```python
from build123d import *

# Parameters (mm, degrees)
F0_R      = 5
F1_DEPTH  = 35
F2_R      = 11.5
F3_DEPTH  = 78
F4_R      = 15
F5_DEPTH  = 25
F6_R      = 5
F7_DEPTH  = 25
F9_W      = 40
F9_H      = 8
F10_DEPTH = 4


with BuildPart() as f1:
    # F0 (on Right) → F1 (new body)
    with BuildSketch(Plane.YZ):
        Circle(F0_R)
    extrude(amount=F1_DEPTH)

    # F2 (on face) → F3 (join)
    with BuildSketch(Plane(origin=(0, 0, 0), x_dir=(0, -1, 0), z_dir=(-1, 0, 0))):
        Circle(F2_R)
    extrude(amount=F3_DEPTH)

    # F4 (on face) → F5 (join)
    with BuildSketch(Plane(origin=(-78, 0, 0), x_dir=(0, -1, 0), z_dir=(-1, 0, 0))):
        Circle(F4_R)
    extrude(amount=F5_DEPTH)

    # F6 (on face) → F7 (join)
    with BuildSketch(Plane(origin=(-103, 0, 0), x_dir=(0, -1, 0), z_dir=(-1, 0, 0))):
        Circle(F6_R)
    extrude(amount=F7_DEPTH)

    # F9 (on offset) → F10 (cut)
    with BuildSketch(Plane.XY.offset(11.5)):
        with Locations((-41.2988585503, 0)):
            Rectangle(F9_W, F9_H)
    extrude(amount=-F10_DEPTH, mode=Mode.SUBTRACT)


solid = f1.part
```
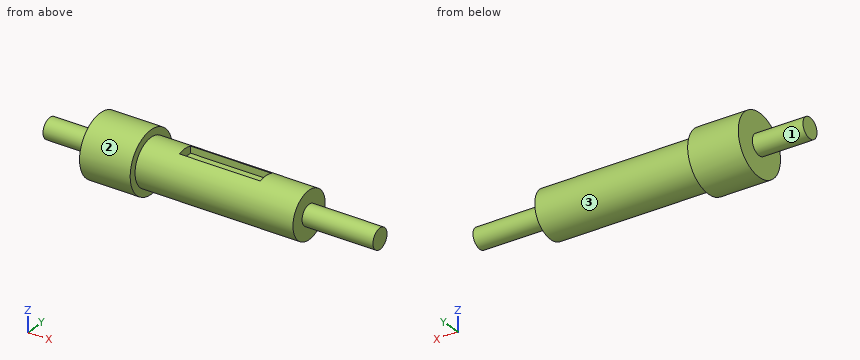
Build history of the part. All positions in model axes, mm. Face numbers are marked on the shaded views. A direction names the side the tool comes from. Round coordinates to 2 decimals unless told otherwise and drop trailing zeros. Write each loop counter-clockwise with the first axis right and the second up, starting at its lowest first coordinate (ties: lowest second). Pieces come first, ordered by that corner, then holes. Notation, with made-up numbers: (65.5, 12.5) - (99.5, 12.5) arc R13 ccw to (99.5, 27.5) - close; hole circle Ø11 at (7, 56). An arc over 180 degrees is marked (long way). Write each question's results on one line, items separated by ' | '. Start each with the question number.
Item 1: Saw through at C-C (x = 3). Write the cut outline in (y, z), and give its area (3 significant figures).
Item 2: Drop flat-ended pins along their axis: P1, Ø12, axis at x = -84, y = -11, coming from the -Z side; P2, Ø3, axis at x = -79.5, z = 11.5, coming from the -Y side; P3, Ø3, axis at y = 0, z = 9, coming from the +X side; P4, Ø15, axis at y = -6.5, z = 0, coming from the +X side. Give the stop position or say it passes through.
Item 3: Wall check: L1, parallel to X at y = -1.25, z = 9.5; L2, parallel to X at y = -8, z = 6; L3, parallel to Z at x = -33.5, y = 0. Give the ranges that are in metal, low to high. Write a range as [from, to].
Item 4: Saw through at B-B (y = 0). Write the cut outline in (x, z).
Item 5: Saw through at D-D (z = -9.25). Write the cut outline in (x, y).
Item 6: Which spindle directions (+Z, -Z, +X, -X, +Y, -Y) get a long thin tool onto all of the face, cutting with end or side? Do the marked faces 1, 2 and 3. Say none if no direction does.
Item 7: Saw through at A-A (z = 0). Write the cut outline in (x, y).
Results are:
1) outline: circle Ø10 at (0, 0) | area: 78.5 mm²
2) P1: stops at z = -14.14 | P2: stops at y = -11.18 | P3: stops at x = 0 | P4: stops at x = 35
3) L1: x = [-103, -61.3], [-21.3, 0] | L2: x = [-103, 0] | L3: z = [-11.5, 7.5]
4) outline: (-128, -5) - (-103, -5) - (-103, -15) - (-78, -15) - (-78, -11.5) - (0, -11.5) - (0, -5) - (35, -5) - (35, 5) - (0, 5) - (0, 11.5) - (-21.3, 11.5) - (-21.3, 7.5) - (-61.3, 7.5) - (-61.3, 11.5) - (-78, 11.5) - (-78, 15) - (-103, 15) - (-103, 5) - (-128, 5) - close
5) outline: (-103, -11.81) - (-78, -11.81) - (-78, -6.83) - (0, -6.83) - (0, 6.83) - (-78, 6.83) - (-78, 11.81) - (-103, 11.81) - close
6) face 1: -X | face 2: +X, -X | face 3: +X
7) outline: (-128, -5) - (-103, -5) - (-103, -15) - (-78, -15) - (-78, -11.5) - (0, -11.5) - (0, -5) - (35, -5) - (35, 5) - (0, 5) - (0, 11.5) - (-78, 11.5) - (-78, 15) - (-103, 15) - (-103, 5) - (-128, 5) - close
